Work out the finished part from the listing and answer in its coordinate system (mm). Face numbers are marked on the shaded views. Give positions to 0.01 mm unless a question says otherwise; leave off trailing zeros. Order: outer loops, then holes, each group sorted by start corner. A loop starts at its lowest first (then second) coordinate and runs counter-clockwise, first axis right, second up.
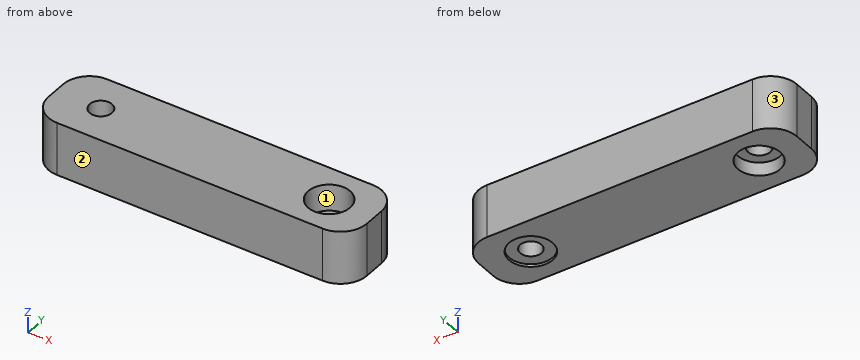
```python
from build123d import *

# Parameters (mm, degrees)
SKETCH1_W           = 60
SKETCH1_H           = 14
BOSS_EXTRUDE1_DEPTH = 10
FILLET1_R           = 5
FILLET2_R           = 5
SKETCH2_R           = 4
CUT_EXTRUDE2_DEPTH  = 2.5
SKETCH3_R           = 2.1
CUT_EXTRUDE3_DEPTH  = 2
SKETCH4_R           = 3.95
CUT_EXTRUDE4_DEPTH  = 5
CUT_EXTRUDE5_REACH  = 64.926
SKETCH5_R           = 2
SKETCH7_R           = 2.1
CUT_EXTRUDE6_DEPTH  = 63.967570185
SKETCH6_R           = 4.1
CUT_EXTRUDE7_DEPTH  = 0.5


with BuildPart() as part:
    # Sketch1 → Boss-Extrude1 (new body)
    with BuildSketch(Plane.XY):
        with Locations((-29.350618243, 13.301945946)):
            Rectangle(SKETCH1_W, SKETCH1_H)
    extrude(amount=BOSS_EXTRUDE1_DEPTH)

    # Fillet1
    fillet1_edges = [part.edges().sort_by_distance(p)[0] for p in [
        (-59.350618243, 20.301945946, 5),
    ]]
    fillet(fillet1_edges, radius=FILLET1_R)

    # Fillet2
    fillet2_edges = [part.edges().sort_by_distance(p)[0] for p in [
        (0.649381757, 20.301945946, 5),
        (0.649381757, 6.301945946, 5),
        (-59.350618243, 6.301945946, 5),
    ]]
    fillet(fillet2_edges, radius=FILLET2_R)

    # Sketch2 → Cut-Extrude2 (cut)
    with BuildSketch(Plane(origin=(0, 0, 0), x_dir=(-1, 0, 0), z_dir=(0, 0, -1))):
        with Locations((50.850618243, 13.301945946)):
            Circle(SKETCH2_R)
    extrude(amount=-CUT_EXTRUDE2_DEPTH, mode=Mode.SUBTRACT)

    # Sketch3 → Cut-Extrude3 (cut)
    with BuildSketch(Plane(origin=(0, 0, 2.5), x_dir=(-1, 0, 0), z_dir=(0, 0, -1))):
        with Locations((50.850618243, 13.301945946)):
            Circle(SKETCH3_R)
    extrude(amount=-CUT_EXTRUDE3_DEPTH, mode=Mode.SUBTRACT)

    # Sketch4 → Cut-Extrude4 (cut)
    with BuildSketch(Plane.XY.offset(10)):
        with Locations((-7.850618243, 13.301945946)):
            Circle(SKETCH4_R)
    extrude(amount=-CUT_EXTRUDE4_DEPTH, mode=Mode.SUBTRACT)

    # Sketch5 → Cut-Extrude5 (cut, up to next)
    with BuildSketch(Plane.XY.offset(5), mode=Mode.PRIVATE) as cut_extrude5_sk1:
        with Locations((-7.850618243, 13.301945946)):
            Circle(SKETCH5_R)
    cut_extrude5_tool1 = extrude(cut_extrude5_sk1.sketch, amount=-CUT_EXTRUDE5_REACH, mode=Mode.PRIVATE) & part.part
    add(cut_extrude5_tool1.solids().sort_by_distance((-7.850618, 13.301946, 5))[0], mode=Mode.SUBTRACT)

    # Sketch7 → Cut-Extrude6 (cut, through all)
    with BuildSketch(Plane(origin=(0, 0, 4.5), x_dir=(-1, 0, 0), z_dir=(0, 0, -1))):
        with Locations((50.850618243, 13.301945946)):
            Circle(SKETCH7_R)
    extrude(amount=-CUT_EXTRUDE6_DEPTH, mode=Mode.SUBTRACT)

    # Sketch6 → Cut-Extrude7 (cut)
    with BuildSketch(Plane(origin=(0, 0, 0), x_dir=(-1, 0, 0), z_dir=(0, 0, -1))):
        with Locations((7.850618243, 13.301945946)):
            Circle(SKETCH6_R)
    extrude(amount=-CUT_EXTRUDE7_DEPTH, mode=Mode.SUBTRACT)


solid = part.part
```
1. Straight lines are drawn through the part: probe 1 along X at (y, z) = (14, 1); probe 2 along X at (y, z) = (14.5, 8.5); probe 3 along X at (y, z) = (15.75, 2.25). For each, find the intervals that lie inside material, in ascending order.
Findings below:
probe 1: x = -59.35 to -54.79, -46.91 to -9.72, -5.98 to 0.65
probe 2: x = -59.35 to -52.58, -49.13 to -11.61, -4.09 to 0.65
probe 3: x = -59.33 to -54.01, -47.69 to 0.63
2. The part is cut by section C-C (y = 10). Write down the section's boundary in (x, z), then the cut area to 3 significant figures.
Findings below:
outline: (-59.18, 0) - (-53.11, 0) - (-53.11, 2.5) - (-48.59, 2.5) - (-48.59, 0) - (-10.28, 0) - (-10.28, 0.5) - (-5.42, 0.5) - (-5.42, 0) - (0.48, 0) - (0.48, 10) - (-5.68, 10) - (-5.68, 5) - (-10.02, 5) - (-10.02, 10) - (-59.18, 10) - close
area: 561 mm2
3. The part is cut by section D-D (z = 4.5). Write down the section's boundary in (x, y), then the cut area to 3 significant figures.
Findings below:
outline: (-59.35, 11.3) arc R5 ccw to (-54.35, 6.3) - (-4.35, 6.3) arc R5 ccw to (0.65, 11.3) - (0.65, 15.3) arc R5 ccw to (-4.35, 20.3) - (-54.35, 20.3) arc R5 ccw to (-59.35, 15.3) - close; hole circle Ø4.2 at (-50.85, 13.3); hole circle Ø4 at (-7.85, 13.3)
area: 792 mm2
4. The part is cut by section A-A (x = -49.5). Write down the section's boundary in (y, z), then the cut area to 3 significant figures.
Findings below:
outline: (6.3, 0) - (9.54, 0) - (9.54, 2.5) - (11.69, 2.5) - (11.69, 10) - (6.3, 10) - close; (14.91, 2.5) - (17.07, 2.5) - (17.07, 0) - (20.3, 0) - (20.3, 10) - (14.91, 10) - close
area: 97.1 mm2
5. The part is cut by section B-B (z = 1). Write down the section's boundary in (x, y), then the cut area to 3 significant figures.
Findings below:
outline: (-59.35, 11.3) arc R5 ccw to (-54.35, 6.3) - (-4.35, 6.3) arc R5 ccw to (0.65, 11.3) - (0.65, 15.3) arc R5 ccw to (-4.35, 20.3) - (-54.35, 20.3) arc R5 ccw to (-59.35, 15.3) - close; hole circle Ø8 at (-50.85, 13.3); hole circle Ø4 at (-7.85, 13.3)
area: 756 mm2
6. The mould has two halves that part along X. Classify the marked faces 1, 2 and 3: pulls with the +X half, pulls with the -X half, needs draft (parallel to the pull), parting line crosses it, or undercut.
Findings below:
face 1: undercut
face 2: needs draft
face 3: pulls with the -X half
7. Given P1, Ø3.5, axis at x = -50.85, y = 13.3, coming from the +Z side (3 decimals); P2, Ø5, axis at x = -7.85, y = 13.3, coming from the -Z side, each flat-ended and moving along its own axis, determine where each tip first touches the part or whether it passes through.
Findings below:
P1: passes through
P2: stops at z = 0.5
